Check sheet for the modelled part. Datum: model origin and axes. Units: mm. A direction names the side the tool comes from. Give positions to 0.01 mm unless a question says otherwise; leave off trailing zeros. Write each loop counter-clockwise with the first axis right and the second up, starting at its lowest first coordinate (ties: lowest second). Pieces come first, ordered by that corner, then holes. Notation, with made-up numbers: (-17, 52) -> (0, 52) arc R22 ccw to (0, 74) -> close; hole circle Ø10 at (9.5, 44). An arc over 180 degrees is marked (long way). Answer as a JSON object with one key per item and string values.
from build123d import *

# Parameters (mm, degrees)
SKIZZE2_W                       = 30
SKIZZE2_H                       = 90
AUFSATZ_LINEAR_AUSTRAGEN2_DEPTH = 2.5
SCHNITT_LINEAR_AUSTRAGEN1_DEPTH = 5
M4_GEWINDEBOHRUNG1_D            = 3.3
M4_GEWINDEBOHRUNG1_DEPTH        = 11.5
M4_GEWINDEBOHRUNG1_TIP          = 0.991420021


with BuildPart() as part:
    # Skizze2 → Aufsatz-Linear austragen2 (new, symmetric)
    with BuildSketch(Plane.XY):
        with Locations((0, 45)):
            Rectangle(SKIZZE2_W, SKIZZE2_H)
    extrude(amount=AUFSATZ_LINEAR_AUSTRAGEN2_DEPTH, both=True)

    # Skizze1 → Schnitt-Linear austragen1 (cut, symmetric)
    with BuildSketch(Plane.XY):
        with BuildLine():
            Line((-11.5, 12.846291202), (-11.5, 15.5))
            ThreePointArc((-11.5, 15.5), (-8, 19), (-4.5, 15.5))
            Line((-4.5, 15.5), (-4.5, 12.846291202))
            ThreePointArc((-4.5, 12.846291202), (-4.25, 11.5), (-4.5, 10.153708798))
            Line((-4.5, 10.153708798), (-4.5, 7.5))
            ThreePointArc((-4.5, 7.5), (-8, 4), (-11.5, 7.5))
            Line((-11.5, 7.5), (-11.5, 10.153708798))
            ThreePointArc((-11.5, 10.153708798), (-11.75, 11.5), (-11.5, 12.846291202))
        make_face()
        with BuildLine():
            Line((4.5, 12.846291202), (4.5, 15.5))
            ThreePointArc((4.5, 15.5), (8, 19), (11.5, 15.5))
            Line((11.5, 15.5), (11.5, 12.846291202))
            ThreePointArc((11.5, 12.846291202), (11.75, 11.5), (11.5, 10.153708798))
            Line((11.5, 10.153708798), (11.5, 7.5))
            ThreePointArc((11.5, 7.5), (8, 4), (4.5, 7.5))
            Line((4.5, 7.5), (4.5, 10.153708798))
            ThreePointArc((4.5, 10.153708798), (4.25, 11.5), (4.5, 12.846291202))
        make_face()
    extrude(amount=SCHNITT_LINEAR_AUSTRAGEN1_DEPTH, both=True, mode=Mode.SUBTRACT)

    # M4 Gewindebohrung1
    with Locations(Plane.XY.offset(2.5)):
        with Locations((-10.5, 82), (10.5, 82)):
            Hole(M4_GEWINDEBOHRUNG1_D / 2, depth=M4_GEWINDEBOHRUNG1_DEPTH)
            with Locations((0, 0, -(M4_GEWINDEBOHRUNG1_DEPTH + M4_GEWINDEBOHRUNG1_TIP / 2))):  # 118° drill point
                Cone(0, M4_GEWINDEBOHRUNG1_D / 2, M4_GEWINDEBOHRUNG1_TIP, mode=Mode.SUBTRACT)


solid = part.part
1. Sectioned sample at C-C, the plane z = 0.8. Enter the section's corners in (x, y), plus the area to 3 significant figures.
Determined:
{"outline": "(-15, 0) -> (15, 0) -> (15, 90) -> (-15, 90) -> close; hole circle Ø3.3 at (-10.5, 82); hole (-11.5, 7.5) arc R3.5 ccw to (-4.5, 7.5) -> (-4.5, 10.15) arc R3.75 ccw to (-4.5, 12.85) -> (-4.5, 15.5) arc R3.5 ccw to (-11.5, 15.5) -> (-11.5, 12.85) arc R3.75 ccw to (-11.5, 10.15) -> close; hole (4.5, 7.5) arc R3.5 ccw to (11.5, 7.5) -> (11.5, 10.15) arc R3.75 ccw to (11.5, 12.85) -> (11.5, 15.5) arc R3.5 ccw to (4.5, 15.5) -> (4.5, 12.85) arc R3.75 ccw to (4.5, 10.15) -> close; hole circle Ø3.3 at (10.5, 82)", "area": "2,490 mm^2"}
2. Mould release check, pull along Y, two halves, no side actions. Record for faces 3 (the face through (0, 0, 0)), 4 (the face through (0, 46, -2.5)), 5 (the face through (4.5, 14, 0)): released by +Y, released by -Y, zero draft, split by the parting line, or undercut.
Determined:
{"face 3": "released by -Y", "face 4": "zero draft", "face 5": "undercut"}
3. Scan lines: L1, parallel to X at y = 82, z = 0.1; L2, parallel to Y at x = 9.5, z = 0.9; L3, parallel to Y at x = -10.5, z = 1.25. Record each from-to range of solid material in increasing order. Write a range as [from, to].
Determined:
{"L1": "[-15, -12.15], [-8.85, 8.85], [12.15, 15]", "L2": "[0, 4.34], [18.66, 80.69], [83.31, 90]", "L3": "[0, 5.05], [17.95, 80.35], [83.65, 90]"}
4. Sectioned sample at B-B, the plane y = 82. Enter the section's corners in (x, z), plus the area to 3 significant figures.
Determined:
{"outline": "(-15, -2.5) -> (-12.15, -2.5) -> (-12.15, 2.5) -> (-15, 2.5) -> close; (-8.85, -2.5) -> (8.85, -2.5) -> (8.85, 2.5) -> (-8.85, 2.5) -> close; (12.15, -2.5) -> (15, -2.5) -> (15, 2.5) -> (12.15, 2.5) -> close", "area": "117 mm^2"}
5. Go/stop test with a flat-tipped pin: P1, Ø1.5, axis at x = -2.5, z = 0, coming from the -Y side. Record where the tip stops, or that it passes through.
Determined:
{"P1": "y = 0"}
6. Access from +Z, -Z, +X, -X, +Y, -Y to the whole of each face (thin tool, end or side, straight path). Record for faces 1 (the face through (15, 44, 0)), 2 (the face through (4.5, 9, 0)).
Determined:
{"face 1": "+Z, -Z, +X, +Y, -Y", "face 2": "+Z, -Z"}
7. Sectioned sample at D-D, the plane y = 17.5. Enter the section's corners in (x, z), plus the area to 3 significant figures.
Determined:
{"outline": "(-15, -2.5) -> (-10.87, -2.5) -> (-10.87, 2.5) -> (-15, 2.5) -> close; (-5.13, -2.5) -> (5.13, -2.5) -> (5.13, 2.5) -> (-5.13, 2.5) -> close; (10.87, -2.5) -> (15, -2.5) -> (15, 2.5) -> (10.87, 2.5) -> close", "area": "92.6 mm^2"}
8. Sectioned sample at A-A, the plane x = 8. Enter the section's corners in (y, z), plus the area to 3 significant figures.
Determined:
{"outline": "(0, -2.5) -> (4, -2.5) -> (4, 2.5) -> (0, 2.5) -> close; (19, -2.5) -> (90, -2.5) -> (90, 2.5) -> (19, 2.5) -> close", "area": "375 mm^2"}
